Study the drawing (mm; zero at the part's minimum x, y, z) and answer. Coordinates: 2 decimals unless noted, no trailing zeros. Order: outer loops, then holes, each group sorted by start corner. A loop starts at its lowest first (then second) coordinate and runs counter-clockwise, first axis right, second up. Notation, with made-up numbers: (45, 15.25) -> (68, 15.25) arc R11 cw to (68, 32.25) -> close; hole circle Ø4 at (31, 89.25). An arc over 180 degrees is marked (long way). Answer as CSV lines item,"result". Start each with the question number.
Item 1: Section A-A (x = 76) is taken. Write down the section's boundary in (y, z).
Item 2: Section D-D (x = 41) is taken. Write down the section's boundary in (y, z), then the cut area to 3 significant figures.
Item 3: Section B-B (y = 26) is taken. Write down the section's boundary in (x, z), then the cut area to 3 significant figures.
Item 4: Straight lines are drawn through the part: L1, parallel to Y at x = 76, z = 1.1; L2, parallel to Z at x = 48.5, y = 33.5; L3, parallel to Z at x = 23, y = 12.5. For each, find the intervals that lie inside material, in ascending order.
Item 5: Each of these flat-tipped pins is pushed along its axis until it touches: pin 1 Ø2 at (x, y) = (4, 31.365) entering from +Z; pin 2 Ø0.6 at (x, z) = (46, 7.5) entering from -Y; pin 3 Ø3 at (x, z) = (24, 4) entering from -Y; pin 4 Ø5.5 at (x, y) = (76, 5.064) entering from +Z. Where does it stop, or does it pass through?
Item 6: Section C-C (x = 4) is taken. Write down the section's boundary in (y, z) (3 decimals), then the cut area to 3 significant figures.
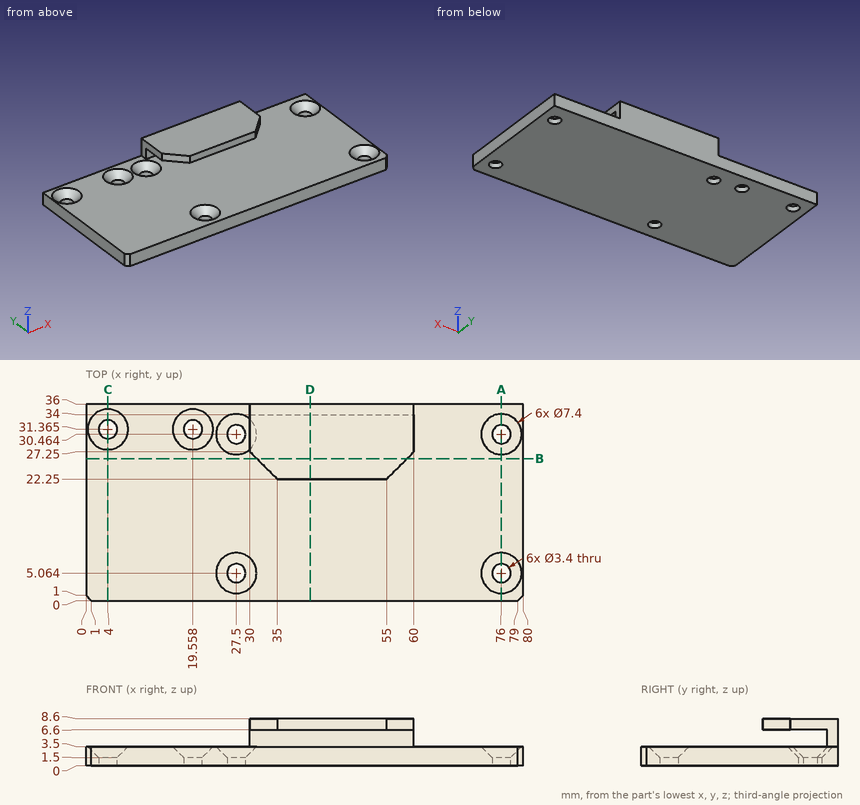
Checked values:
1,outline,"(0, 0) -> (3.36, 0) -> (3.36, 1.5) -> (1.36, 3.5) -> (0, 3.5) -> close; (6.76, 0) -> (28.76, 0) -> (28.76, 1.5) -> (26.76, 3.5) -> (8.76, 3.5) -> (6.76, 1.5) -> close; (32.16, 0) -> (36, 0) -> (36, 3.5) -> (34.16, 3.5) -> (32.16, 1.5) -> close"
2,outline,"(0, 0) -> (36, 0) -> (36, 8.6) -> (22.25, 8.6) -> (22.25, 6.6) -> (34, 6.6) -> (34, 3.5) -> (0, 3.5) -> close"
2,area,"160 mm^2"
3,outline,"(0, 0) -> (80, 0) -> (80, 3.5) -> (0, 3.5) -> close; (31.25, 6.6) -> (58.75, 6.6) -> (58.75, 8.6) -> (31.25, 8.6) -> close"
3,area,"335 mm^2"
4,L1,"y = 0 to 3.36, 6.76 to 28.76, 32.16 to 36"
4,L2,"z = 0 to 3.5, 6.6 to 8.6"
4,L3,"z = 0 to 3.5"
5,pin 1,"passes through"
5,pin 2,"stops at y = 22.25"
5,pin 3,"stops at y = 0"
5,pin 4,"stops at z = 2.55"
6,outline,"(0, 0) -> (29.665, 0) -> (29.665, 1.5) -> (27.665, 3.5) -> (0, 3.5) -> close; (33.065, 0) -> (36, 0) -> (36, 3.5) -> (35.065, 3.5) -> (33.065, 1.5) -> close"
6,area,"110 mm^2"
